Autodesk Inventor part; units mm, degrees
ref_plane "XZ Plane" through (0, 0, 0) normal (0, 1, 0) x (-1, 0, 0)
ref_plane "XY Plane" through (0, 0, 0) normal (0, 0, 1) x (1, 0, 0)
sketch "Sketch1" plane through (0, 0, 0) normal (0, 0, 1) x (1, 0, 0)
  line L0 (-12, 0) -> (12, 0) construction
  line L1 (-12, -4) -> (12, -4)
  line L2 (12, 4) -> (-12, 4)
  arc A0 (-12, 4) -> (-12, -4) centre (-12, 0) ccw
  arc A1 (12, -4) -> (12, 4) centre (12, 0) ccw
  point P0 (0, 0)
  dimension "d0" = 24
  dimension "d1" = 4
extrude "Extrusion1" add sketch "Sketch1" along normal blind 4
sketch "Sketch2" plane through (0, 0, 4) normal (0, 0, 1) x (1, 0, 0)
  circle A0 centre (0, 0) radius 3
  dimension "d4" = 6
extrude "Extrusion2" add sketch "Sketch2" along normal blind 16
chamfer "Chamfer1" distance 0.5 angle 45 1 edges at (-3, 0, 20)
sketch "Sketch3" plane through (0, 0, 4) normal (0, 0, 1) x (1, 0, 0)
  arc A0 (12, -4) -> (12, 4) centre (12, 0) ccw
  arc A1 (-12, 4) -> (-12, -4) centre (-12, 0) ccw
hole "Hole1" at (-12, 0, 4) at (12, 0, 4) direction (0, 0, -1) diameter 4 end through all
ref_plane "Work Plane1" through (0, 0, 15) normal (0, 0, 1) x (1, 0, 0)
hole "Hole2" at (0, 3, 15) direction (0, -1, 0) diameter 2 end through all
properties part number "Crank" material "Steel"
Verification items for the finished model (mm, model axes). A direction names the side the tool comes from. Coordinates: 2 decimals unless noted, no trailing zeros. Loops run counter-clockwise (first coordinate to the right, second up) from the corner with the lowest first, then second, coordinate; pieces in that order, holes last. Notation, with made-up numbers: (5, -24.5) -> (39, -24.5) arc R37 cw to (39, 14.5) -> close; hole circle Ø8 at (85.5, 41). An arc over 180 degrees is marked (long way). Write each question's results on one line, items separated by ' | '.
Item 1: Material ranges on L1, parallel to X at y = 0, z = 1.25; L2, parallel to Y at x = -12, z = 1.2; L3, parallel to Z at x = 2, y = -3, recorded low to high.
Found:
L1: x = -16 to -14, -10 to 10, 14 to 16 | L2: y = -4 to -2, 2 to 4 | L3: z = 0 to 4
Item 2: Gauge pin test, flat ends, axial feed: pin 1 (4 mm diameter, centred on x = 3.5, y = 1.5, fed in from +Z); pin 2 (5 mm diameter, centred on x = 6.5, z = 10, fed in from +Y); pin 3 (4 mm diameter, centred on y = 2, z = 12, fed in from +X); pin 4 (2.5 mm diameter, centred on x = 0, z = 15, fed in from -Y). Record the tip position at first contact, or that the pin passes through.
Found:
pin 1: stops at z = 20 | pin 2: passes through | pin 3: stops at x = 3 | pin 4: stops at y = -3
Item 3: Section check C-C, the plane z = 3.5. Enter the section's corners in (x, y).
Found:
outline: (-12, -4) -> (12, -4) arc R4 ccw to (12, 4) -> (-12, 4) arc R4 ccw to start; hole circle Ø4 at (-12, 0); hole circle Ø4 at (12, 0)
Item 4: Tool access check on faces 4 (the face through (2.77, 1.15, 11.64)), 5 (the face through (0, 4, 2)). Record the directions out of +Z, -Z, +X, -X, +Y, -Y that give a thin tool (end or side, any length) a straight path to the whole face; none if there is none.
Found:
face 4: +Z | face 5: +Z, -Z, +X, -X, +Y
Item 5: Mould release check, pull along X, two halves, no side actions. Record for faces 1 (the face through (16, 0, 2)), 2 (the face through (-14, 0, 2)), 3 (the face through (0, 0, 20)): +X half, -X half, draft (parallel to the pull), parting line (faces both ways), or undercut.
Found:
face 1: +X half | face 2: undercut | face 3: draft
Item 6: Section check D-D, the plane z = 15. Enter the section's corners in (x, y), plus the area to 3 significant figures.
Found:
outline: (-1, -2.83) -> (-1, 2.83) arc R3 ccw to start; (1, -2.83) arc R3 ccw to (1, 2.83) -> close | area: 16.5 mm2
Item 7: Section check A-A, the plane y = 0. Enter the section's corners in (x, z).
Found:
outline: (-16, 0) -> (-14, 0) -> (-14, 4) -> (-16, 4) -> close; (-10, 0) -> (10, 0) -> (10, 4) -> (3, 4) -> (3, 19.5) -> (2.5, 20) -> (-2.5, 20) -> (-3, 19.5) -> (-3, 4) -> (-10, 4) -> close; (14, 0) -> (16, 0) -> (16, 4) -> (14, 4) -> close; hole circle Ø2 at (0, 15)
Item 8: Section check B-B, the plane x = 0. Enter the section's corners in (y, z), plus the area to 3 significant figures.
Found:
outline: (-4, 0) -> (4, 0) -> (4, 4) -> (3, 4) -> (3, 14) -> (-3, 14) -> (-3, 4) -> (-4, 4) -> close; (-3, 16) -> (3, 16) -> (3, 19.5) -> (2.5, 20) -> (-2.5, 20) -> (-3, 19.5) -> close | area: 116 mm2
